Part model, mm, in its own coordinate system. A direction names the side the tool comes from. Coordinates: 2 decimals unless noted, no trailing zeros. Write each loop counter-clockwise with the first axis right and the second up, starting at its lowest first coordinate (ties: lowest second). Pieces come first, ordered by that corner, then holes. Notation, with made-up numbers: (-2, 63) -> (14, 63) arc R22 ccw to (14, 98) -> close; hole circle Ø2 at (13.25, -37.5). An arc over 180 degrees is marked (long way). One line per question, with ' | ' between items. Start each with the question number.
Item 1: Two-plate mould, pull along Y, no slides. Class faces 1 (the cylindrical face through (6.41, 20.08, 0.54)), 2 (the cylindrical face through (-0.03, -35.43, 0.54)), 3 (the cylindrical face through (0.1, -26.45, 4.47)): pulls with the +Y half, pulls with the -Y half, needs draft (parallel to the pull), parting line crosses it, or undercut.
Item 2: Pin check, flat tips, straight feed: pin 1 (5.5 mm diameter, centred on x = 6.5, z = 6.5, fed in from +Y); pin 2 (5 mm diameter, centred on x = 9, y = 16, fed in from -Z); pin 3 (3.5 mm diameter, centred on y = 0, z = 5.08, fed in from +X). Stop position of each tip, or through.
Item 3: 3-axis set-ups, long thin cutter, end or side, ignore diameter. For faces 4 (the cylindrical face through (6.41, 20.08, 9.62)), 5 (the cylindrical face through (6.41, -20.38, 0.54)), 6 (the cylindrical face through (-6.41, -20.08, 9.62)): which of +Z, -Z, +X, -X, +Y, -Y reach the whole face in a straight line?
Item 4: Saw through at D-D (y = 14). List the corners of the cut face in (x, z) (3 decimals).
Item 5: Saw through at A-A (y = 0). List the corners of the cut face in (x, z) (3 decimals), and give its area (3 significant figures).
Item 6: Saw through at C-C (z = 9). List the corners of the cut face in (x, y) (3 decimals).
Item 7: Probe probe 1 along Y at (x, z) = (1.25, 4.5); probe 2 along Y at (x, z) = (-5, 4.5); probe 3 along Y at (x, z) = (-3.75, 4.75). List the from-to ranges inside material, lowest first. Write a range as [from, to].
Item 8: Saw through at B-B (z = 5.08). Count the separate pieces of the cut face and the enclosed holes in it, and give its area (3 significant figures).
from build123d import *

# Parameters (mm, degrees)
SKETCH2_R           = 2.032
BOSS_EXTRUDE1_DEPTH = 10.16
SKETCH3_W           = 6.38
SKETCH3_H           = 6.38
CUT_EXTRUDE1_DEPTH  = 40.509368553
SKETCH4_R           = 2.032
CUT_EXTRUDE2_DEPTH  = 24.13
FILLET3_R           = 1.905
FILLET1_R           = 5.08
SKETCH5_R           = 2.032
CUT_EXTRUDE3_DEPTH  = 41.64716852
SKETCH7_W           = 10.16
SKETCH7_H           = 8.636
CUT_EXTRUDE4_DEPTH  = 5.842
SKETCH8_W           = 10.16
SKETCH8_H           = 8.636
BOSS_EXTRUDE2_DEPTH = 1.016


with BuildPart() as part:
    # Sketch2 → Boss-Extrude1 (new body)
    with BuildSketch(Plane.XY):
        with BuildLine():
            Line((-6.985, 10.606591111), (-6.985, 36.006591111))
            Line((-6.985, 36.006591111), (6.985, 36.006591111))
            Line((6.985, 36.006591111), (6.985, 10.606591111))
            ThreePointArc((6.985, 10.606591111), (12.7, 0), (6.985, -10.606591111))
            Line((6.985, -10.606591111), (6.985, -36.006591111))
            Line((6.985, -36.006591111), (-6.985, -36.006591111))
            Line((-6.985, -36.006591111), (-6.985, -10.606591111))
            ThreePointArc((-6.985, -10.606591111), (-12.7, 0), (-6.985, 10.606591111))
        make_face()
        Circle(SKETCH2_R, mode=Mode.SUBTRACT)
    extrude(amount=BOSS_EXTRUDE1_DEPTH)

    # Sketch3 → Cut-Extrude1 (cut, through all)
    with BuildSketch(Plane(origin=(0, 0, 0), x_dir=(-1, 0, 0), z_dir=(0, 0, -1))):
        Rectangle(SKETCH3_W, SKETCH3_H)
    extrude(amount=-CUT_EXTRUDE1_DEPTH, mode=Mode.SUBTRACT)

    # Sketch4 → Cut-Extrude2 (cut)
    with BuildSketch(Plane(origin=(6.985, 0, 3.175), x_dir=(0, 0, 1), z_dir=(-1, 0, 0))):
        with Locations(Location((1.905, 28.386591111, 0), (0, 0, 90))):
            Circle(SKETCH4_R)
        with Locations(Location((1.905, -28.386591111, 0), (0, 0, 90))):
            Circle(SKETCH4_R)
    extrude(amount=CUT_EXTRUDE2_DEPTH, mode=Mode.SUBTRACT)

    # Fillet3
    fillet3_edges = [part.edges().sort_by_distance(p)[0] for p in [
        (6.985, 23.306591111, 0),
        (12.7, 0, 0),
        (6.985, -23.306591111, 0),
        (0, -36.006591111, 0),
        (12.7, 0, 10.16),
        (6.985, 23.306591111, 10.16),
        (0, 36.006591111, 10.16),
        (-6.985, 23.306591111, 10.16),
        (-12.7, 0, 10.16),
        (-6.985, -23.306591111, 10.16),
        (0, -36.006591111, 10.16),
        (-6.985, -23.306591111, 0),
        (6.985, -23.306591111, 10.16),
        (-12.7, 0, 0),
        (-6.985, 23.306591111, 0),
        (0, 36.006591111, 0),
    ]]
    fillet(fillet3_edges, radius=FILLET3_R)

    # Fillet1
    # the kernel refuses this fillet: 5.08 mm, written as the material it takes off along each edge
    with BuildSketch(Plane(origin=(-1.905, 30.926591111, 0), x_dir=(-1, 0, 0), z_dir=(0, -1, 0))) as fillet1_piece_1:
        with BuildLine():
            CenterArc((3.175, -1.905), 1.905, 0, 90)
            Line((5.08, -1.905), (5.08, 0))
            Line((5.08, 0), (3.175, 0))
        make_face()
    revolve(axis=Axis((-1.905, 30.926591111, 0), (0, 0, -1)), revolution_arc=90, mode=Mode.SUBTRACT)
    with BuildSketch(Plane(origin=(1.905, 30.926591111, 0), x_dir=(0, 1, 0), z_dir=(-1, 0, 0))) as fillet1_piece_2:
        with BuildLine():
            CenterArc((3.175, -1.905), 1.905, 0, 90)
            Line((5.08, -1.905), (5.08, 0))
            Line((5.08, 0), (3.175, 0))
        make_face()
    revolve(axis=Axis((1.905, 30.926591111, 0), (0, 0, -1)), revolution_arc=90, mode=Mode.SUBTRACT)
    with BuildSketch(Plane(origin=(-1.905, -30.926591111, 0), x_dir=(0, -1, 0), z_dir=(1, 0, 0))) as fillet1_piece_3:
        with BuildLine():
            CenterArc((3.175, -1.905), 1.905, 0, 90)
            Line((5.08, -1.905), (5.08, 0))
            Line((5.08, 0), (3.175, 0))
        make_face()
    revolve(axis=Axis((-1.905, -30.926591111, 0), (0, 0, -1)), revolution_arc=90, mode=Mode.SUBTRACT)
    with BuildSketch(Plane(origin=(1.905, -30.926591111, 0), x_dir=(1, 0, 0), z_dir=(0, 1, 0))) as fillet1_piece_4:
        with BuildLine():
            CenterArc((3.175, -1.905), 1.905, 0, 90)
            Line((5.08, -1.905), (5.08, 0))
            Line((5.08, 0), (3.175, 0))
        make_face()
    revolve(axis=Axis((1.905, -30.926591111, 0), (0, 0, -1)), revolution_arc=90, mode=Mode.SUBTRACT)
    with BuildSketch(Plane(origin=(-1.905, 30.926591111, 10.16), x_dir=(0, 1, 0), z_dir=(1, 0, 0))) as fillet1_piece_5:
        with BuildLine():
            CenterArc((3.175, -1.905), 1.905, 0, 90)
            Line((5.08, -1.905), (5.08, 0))
            Line((5.08, 0), (3.175, 0))
        make_face()
    revolve(axis=Axis((-1.905, 30.926591111, 10.16), (0, 0, 1)), revolution_arc=90, mode=Mode.SUBTRACT)
    with BuildSketch(Plane(origin=(1.905, 30.926591111, 10.16), x_dir=(1, 0, 0), z_dir=(0, -1, 0))) as fillet1_piece_6:
        with BuildLine():
            CenterArc((3.175, -1.905), 1.905, 0, 90)
            Line((5.08, -1.905), (5.08, 0))
            Line((5.08, 0), (3.175, 0))
        make_face()
    revolve(axis=Axis((1.905, 30.926591111, 10.16), (0, 0, 1)), revolution_arc=90, mode=Mode.SUBTRACT)
    with BuildSketch(Plane(origin=(-1.905, -30.926591111, 10.16), x_dir=(-1, 0, 0), z_dir=(0, 1, 0))) as fillet1_piece_7:
        with BuildLine():
            CenterArc((3.175, -1.905), 1.905, 0, 90)
            Line((5.08, -1.905), (5.08, 0))
            Line((5.08, 0), (3.175, 0))
        make_face()
    revolve(axis=Axis((-1.905, -30.926591111, 10.16), (0, 0, 1)), revolution_arc=90, mode=Mode.SUBTRACT)
    with BuildSketch(Plane(origin=(1.905, -30.926591111, 10.16), x_dir=(0, -1, 0), z_dir=(-1, 0, 0))) as fillet1_piece_8:
        with BuildLine():
            CenterArc((3.175, -1.905), 1.905, 0, 90)
            Line((5.08, -1.905), (5.08, 0))
            Line((5.08, 0), (3.175, 0))
        make_face()
    revolve(axis=Axis((1.905, -30.926591111, 10.16), (0, 0, 1)), revolution_arc=90, mode=Mode.SUBTRACT)
    with BuildSketch(Plane(origin=(6.985, -36.006591111, 0), x_dir=(-1, 0, 0), z_dir=(0, 0, 1)), Plane(origin=(-6.985, -36.006591111, 0), x_dir=(0, 1, 0), z_dir=(0, 0, 1))) as fillet1_piece_9:
        with BuildLine():
            CenterArc((FILLET1_R, -FILLET1_R), FILLET1_R, 90, 90)
            Line((0, -FILLET1_R), (0, 0))
            Line((0, 0), (FILLET1_R, 0))
        make_face()
    extrude(amount=10.16, mode=Mode.SUBTRACT)
    with BuildSketch(Plane(origin=(-6.985, 36.006591111, 0), x_dir=(0, -1, 0), z_dir=(0, 0, 1)), Plane(origin=(6.985, 36.006591111, 0), x_dir=(-1, 0, 0), z_dir=(0, 0, 1))) as fillet1_piece_10:
        with BuildLine():
            CenterArc((FILLET1_R, FILLET1_R), FILLET1_R, 180, 90)
            Line((0, FILLET1_R), (0, 0))
            Line((0, 0), (FILLET1_R, 0))
        make_face()
    extrude(amount=10.16, mode=Mode.SUBTRACT)

    # Sketch5 → Cut-Extrude3 (cut, through all)
    with BuildSketch(Plane.ZY.offset(-3.19)):
        with Locations(Location((5.08, 0, 0), (0, 0, 270))):
            Circle(SKETCH5_R)
    extrude(amount=-CUT_EXTRUDE3_DEPTH, mode=Mode.SUBTRACT)

    # Sketch7 → Cut-Extrude4 (cut)
    with BuildSketch(Plane.ZY.offset(-3.19)):
        with Locations((5.08, 0)):
            Rectangle(SKETCH7_W, SKETCH7_H)
    extrude(amount=-CUT_EXTRUDE4_DEPTH, mode=Mode.SUBTRACT)

    # Sketch8 → Boss-Extrude2 (add)
    with BuildSketch(Plane(origin=(3.19, 0, 0), x_dir=(0, 0, -1), z_dir=(1, 0, 0))):
        with Locations((-5.08, 0)):
            Rectangle(SKETCH8_W, SKETCH8_H)
    extrude(amount=BOSS_EXTRUDE2_DEPTH)


solid = part.part
From the geometry:
1) face 1: needs draft | face 2: pulls with the -Y half | face 3: undercut
2) pin 1: y = 35.66 | pin 2: z = 0.64 | pin 3: x = 4.21
3) face 4: +Z, +X, +Y | face 5: -Z, +X, -Y | face 6: +Z, -X, -Y
4) outline: (-6.985, 1.905) arc R1.905 ccw to (-5.08, 0) -> (5.08, 0) arc R1.905 ccw to (6.985, 1.905) -> (6.985, 8.255) arc R1.905 ccw to (5.08, 10.16) -> (-5.08, 10.16) arc R1.905 ccw to (-6.985, 8.255) -> close
5) outline: (-12.7, 1.905) arc R1.905 ccw to (-10.795, 0) -> (-3.19, 0) -> (-3.19, 10.16) -> (-10.795, 10.16) arc R1.905 ccw to (-12.7, 8.255) -> close; (3.19, 0) -> (4.206, 0) -> (4.206, 10.16) -> (3.19, 10.16) -> close; (9.032, 0) -> (10.795, 0) arc R1.905 ccw to (12.7, 1.905) -> (12.7, 3.048) -> (9.032, 3.048) -> close; (9.032, 7.112) -> (12.7, 7.112) -> (12.7, 8.255) arc R1.905 ccw to (10.795, 10.16) -> (9.032, 10.16) -> close | area: 126 mm2
6) outline: (-6.833, -30.927) arc R4.928 ccw to (-1.905, -35.855) -> (1.905, -35.855) arc R4.928 ccw to (6.833, -30.927) -> (6.833, -10.525) arc R12.548 ccw to (6.833, 10.525) -> (6.833, 30.927) arc R4.928 ccw to (1.905, 35.855) -> (-1.905, 35.855) arc R4.928 ccw to (-6.833, 30.927) -> (-6.833, 10.525) arc R12.548 ccw to (-6.833, -10.525) -> close; hole (-3.19, -3.19) -> (3.19, -3.19) -> (3.19, 3.19) -> (-3.19, 3.19) -> close; hole (4.206, -4.318) -> (9.032, -4.318) -> (9.032, 4.318) -> (4.206, 4.318) -> close
7) probe 1: [-36.01, -30.33], [-26.44, -3.19], [3.19, 26.44], [30.33, 36.01] | probe 2: [-34.95, -30.33], [-26.44, 26.44], [30.33, 34.95] | probe 3: [-35.66, -30.39], [-26.38, 26.38], [30.39, 35.66]
8) separate pieces: 3 | enclosed holes: 1 | area: 944 mm2
